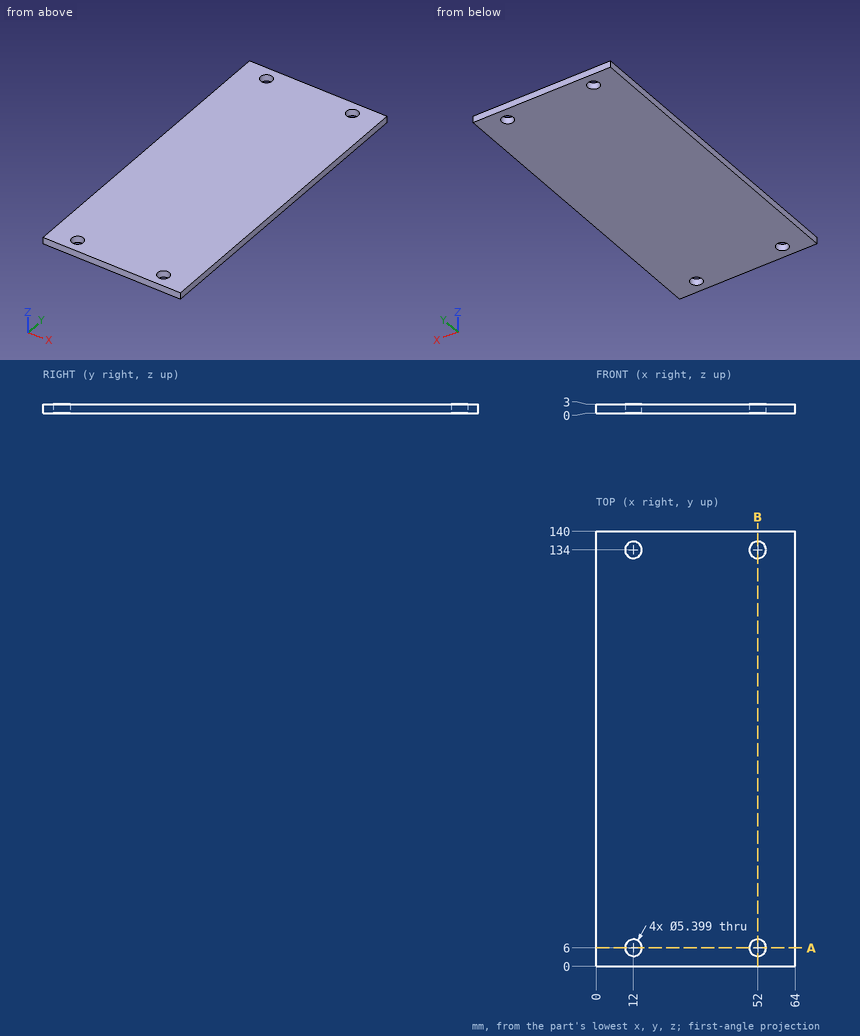
Input: dimensioned drawing with shaded views. Units: mm. Origin: part minimum x, y, z. Coordinates: 2 decimals unless noted, no trailing zeros. Order: outer loops, then holes, each group sorted by start corner. A loop starts at its lowest first (then second) coordinate and runs counter-clockwise, first axis right, second up. Notation, with made-up numbers: M 71,-34 L 117,-34 A30 ccw 117,-10 Z; hole C -10,2 d9. An arc over 180 degrees is marked long. Answer as CSV lines item,"result".
Q1. Section B-B on x = 52. Return the cut outline in (y, z).
Answers:
outline,"M 0,0 L 3.3,0 L 3.3,3 L 0,3 Z; M 8.7,0 L 131.3,0 L 131.3,3 L 8.7,3 Z; M 136.7,0 L 140,0 L 140,3 L 136.7,3 Z"
Q2. First-contact query: P1, Ø6, axis at x = 34, y = 102.5, coming from the -Z side. Flat tip, straight axial feed; report the tip coordinate or a pass-through.
Answers:
P1,"stops at z = 0"
Q3. Section A-A on y = 6. Return the cut outline in (x, z).
Answers:
outline,"M 0,0 L 9.3,0 L 9.3,3 L 0,3 Z; M 14.7,0 L 49.3,0 L 49.3,3 L 14.7,3 Z; M 54.7,0 L 64,0 L 64,3 L 54.7,3 Z"
Q4. Line query: probe 1 along X at (y, z) = (134, 1.35); probe 2 along Y at (x, z) = (12, 1.3); probe 3 along Y at (x, z) = (10.5, 0.55) (1 decimal). Output: solid intervals per line, ascending. Write a range as [from, to].
Answers:
probe 1,"x = [0, 9.3], [14.7, 49.3], [54.7, 64]"
probe 2,"y = [0, 3.3], [8.7, 131.3], [136.7, 140]"
probe 3,"y = [0, 3.8], [8.2, 131.8], [136.2, 140]"
